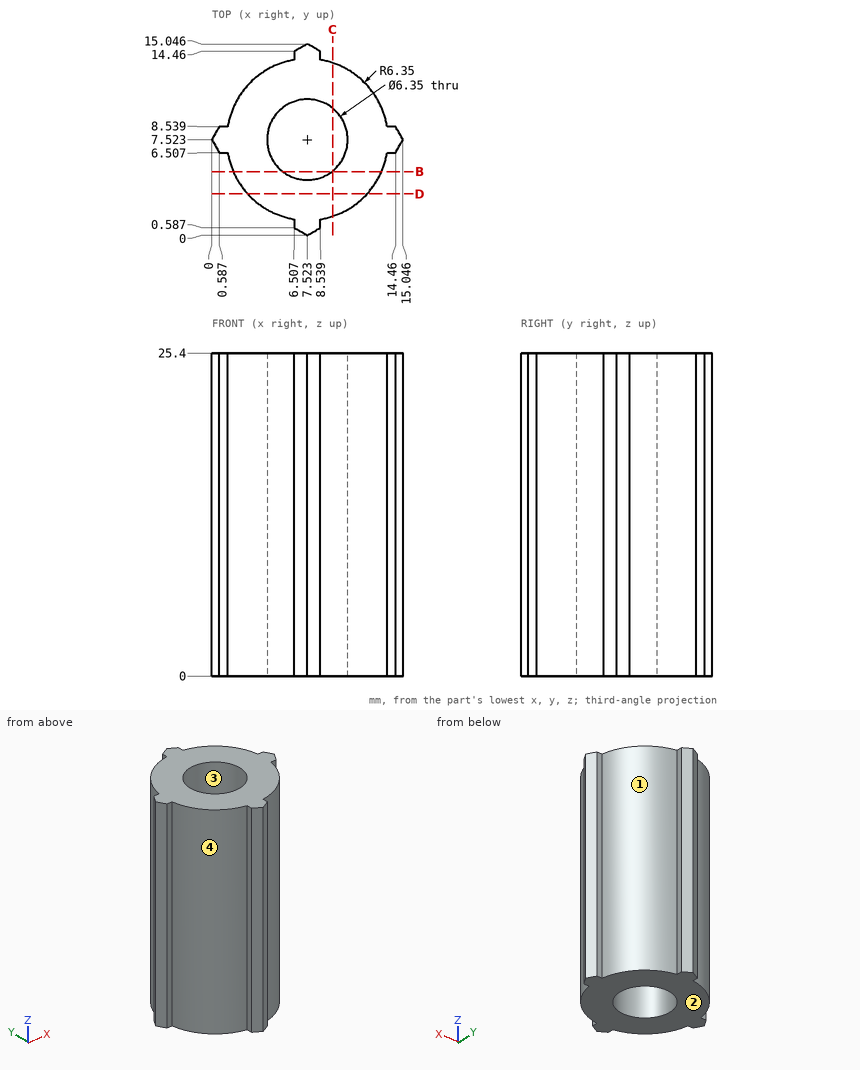
Geometry check sheet. Reference: drawing and pictorial views, mm from the part's lowest x, y, z. Round coordinates to 2 decimals unless told otherwise and drop trailing zeros. Loops run counter-clockwise (first coordinate to the right, second up) from the corner with the lowest first, then second, coordinate; pieces in that order, holes last.
1. Mould release check, pull along Y, two halves, no side actions. Record for the marked faces 1, 2, 3 and 4: released by +Y, released by -Y, zero draft, split by the parting line, or undercut.
2. Sectioned sample at C-C on x = 9.5. Record the boundary of the cut face in (y, z).
3. Scan lines: probe 1 along X at (y, z) = (10, 11.5) (1 decimal); probe 2 along Y at (x, z) = (8, 11) (1 decimal). Record each from-to range of solid material in increasing order.
4. Sectioned sample at D-D on y = 3.25. Record the boundary of the cut face in (x, z).
5. Gauge pin test, flat ends, axial feed: pin 1 Ø8 at (x, z) = (7.5, 21) entering from -Y; pin 2 Ø3 at (x, y) = (11, 1.5) entering from +Z; pin 3 Ø1.5 at (x, z) = (5, 7.5) entering from +Y; pin 4 Ø5.5 at (x, y) = (7.52, 7.52) entering from -Z. Record the tip position at first contact, or that the pin passes through.
6. Sectioned sample at B-B on y = 5. Record the boundary of the cut face in (x, z), and give its area (3 significant figures).
Recorded:
1. face 1: released by +Y
1. face 2: zero draft
1. face 3: undercut
1. face 4: released by -Y
2. outline: (1.49, 0) - (5.04, 0) - (5.04, 25.4) - (1.49, 25.4) - close; (10.01, 0) - (13.56, 0) - (13.56, 25.4) - (10.01, 25.4) - close
3. probe 1: x = 1.7 to 5.5, 9.5 to 13.4
3. probe 2: y = 0.3 to 4.4, 10.7 to 14.8
4. outline: (2.83, 0) - (12.22, 0) - (12.22, 25.4) - (2.83, 25.4) - close
5. pin 1: stops at y = 0
5. pin 2: stops at z = 25.4
5. pin 3: stops at y = 13.62
5. pin 4: passes through
6. outline: (1.7, 0) - (5.6, 0) - (5.6, 25.4) - (1.7, 25.4) - close; (9.45, 0) - (13.35, 0) - (13.35, 25.4) - (9.45, 25.4) - close
6. area: 198 mm2
